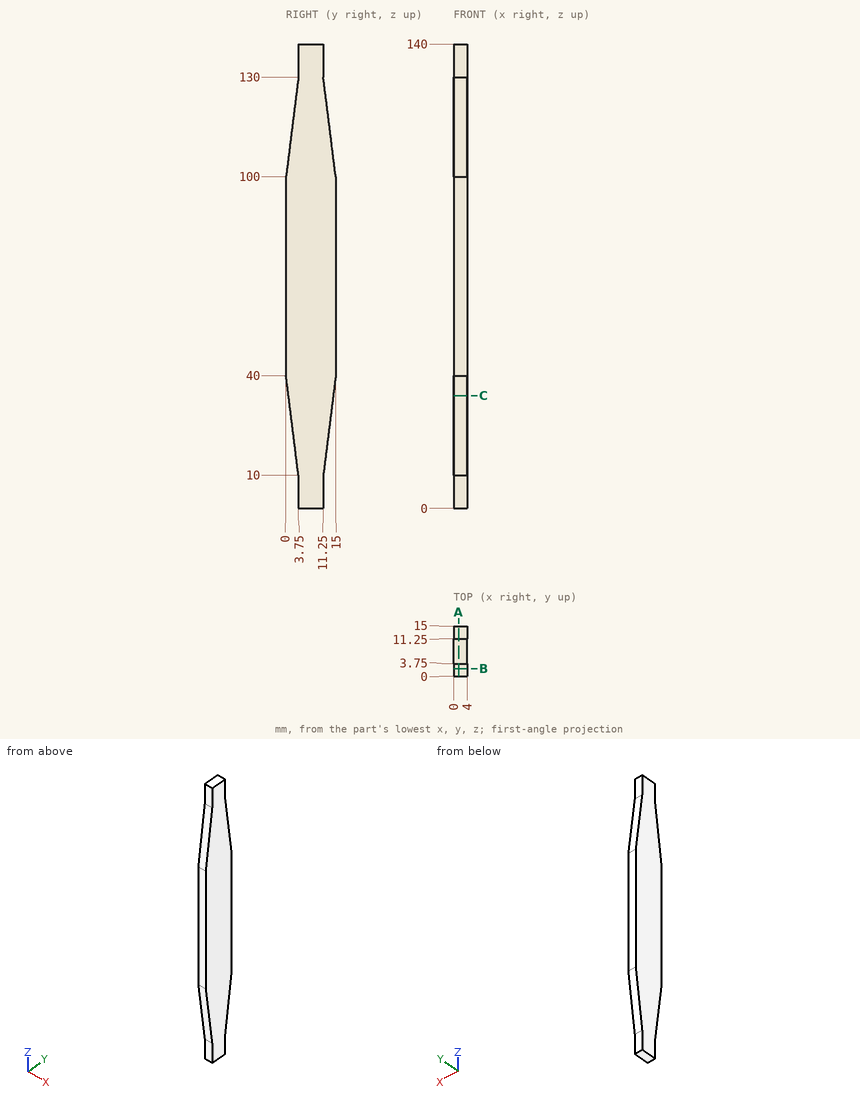
Answer from the drawing. Dimensions are ordinates in mm from the lowest x, y and z of the part. Round coordinates to 2 decimals unless told otherwise and drop trailing zeros. Write each loop counter-clockwise with the first axis right and the second up, starting at its lowest first coordinate (ties: lowest second). Pieces come first, ordered by that corner, then holes. Notation, with made-up numbers: (17.25, 37.5) -> (38.25, 37.5) arc R27 cw to (38.25, 65.5) -> close; hole circle Ø1 at (13, 39.25). An arc over 180 degrees is marked (long way). Answer in a Markdown table with one row per item. Add a question column.
1) Find section B-B, the plane y = 2.25. Determine the outline of the cut face in (x, z), and give its area (3 significant figures).
2) Given P1, Ø2, axis at x = 1.5, z = 2.5, coming from the -Y side; P2, Ø2, axis at x = 2.5, z = 135, coming from the +Y side, each flat-ended and moving along its own axis, determine where each tip first touches the part or whether it passes through.
3) Find section A-A, the plane x = 1.5. Determine the outline of the cut face in (y, z).
4) Consider line 1 (Y direction, x = 2.95, z = 9); line 2 (Y direction, x = 3.65, z = 121.5). Determine where each line is inside the solid, lowest interval first.
5) Find section C-C, the plane z = 34. Determine the outline of the cut face in (x, y).
Findings below:
| question | item | result |
|---|---|---|
| 1 | outline | (0, 22) -> (4, 22) -> (4, 118) -> (0, 118) -> close |
| 1 | area | 384 mm² |
| 2 | P1 | y = 3.75 |
| 2 | P2 | y = 11.25 |
| 3 | outline | (0, 40) -> (3.75, 10) -> (3.75, 0) -> (11.25, 0) -> (11.25, 10) -> (15, 40) -> (15, 100) -> (11.25, 130) -> (11.25, 140) -> (3.75, 140) -> (3.75, 130) -> (0, 100) -> close |
| 4 | line 1 | 3.75 to 11.25 |
| 4 | line 2 | 2.69 to 12.31 |
| 5 | outline | (0, 0.75) -> (4, 0.75) -> (4, 14.25) -> (0, 14.25) -> close |
